For this review, take the finished solid that the model builds, in its own axes (mm). Face numbers are marked on the shaded views. Coordinates: 2 decimals unless noted, no trailing zeros. Loops run counter-clockwise (first coordinate to the right, second up) from the corner with the lowest first, then second, coordinate; pieces in that order, holes last. Notation, with made-up numbers: (22, 13) - (60, 13) arc R19 cw to (60, 35) - close; hole circle Ø3 at (28, 32). An arc over 180 degrees is marked (long way). One line per item, written item: value. Start each with the question number.
1. Take a section at A-A, the plane z = -22.85. State the section outline as (x, y) points (3 decimals), and give its area (3 significant figures).
2. To check wall thickness, follow line 1 (Z direction, x = 5, y = 16.75); line 2 (Z direction, x = 52.95, y = 0.7) (3 decimals); line 3 (X direction, y = 0.7, z = -22.85) (3 decimals). State the ranges of each line that lie inside material, in increasing order. Write a range as from..to.
3. Take a section at B-B, the plane y = 8.5. State the section outline as (x, z) points, and give its area (3 significant figures).
4. The part is to be moulded in two halves that separate along Z. For the marked faces 1, 2, 3 and 4, say which applies: released by +Z, released by -Z, zero draft, split by the parting line, or undercut.
5. Take a section at C-C, the plane x = 7. State the section outline as (y, z) points, and give its area (3 significant figures).
6. Insertion check: pin 1 (2.5 mm diameter, centred on x = 52.95, z = -22.85, fed in from +Y). The pin has a flat end and moves straight along its axis. Give the tip position at first contact, or say it passes through.
```python
from build123d import *

# Parameters (mm, degrees)
SKETCH1_R           = 2.225
BASEPLATE_DEPTH     = 1
BOSS_EXTRUDE4_DEPTH = 21.9


with BuildPart() as part:
    # Sketch1 → BasePlate (new body)
    with BuildSketch(Plane(origin=(0, 0, 0), x_dir=(1, 0, 0), z_dir=(0, 1, 0))):
        with BuildLine():
            Line((5.45, 25.1), (0, 25.1))
            Line((0, 25.1), (0, 45.7))
            Line((0, 45.7), (58.4, 45.7))
            Line((58.4, 45.7), (58.4, 0))
            Line((58.4, 0), (0, 0))
            Line((0, 0), (0, 20.6))
            Line((0, 20.6), (5.45, 20.6))
            ThreePointArc((5.45, 20.6), (7.7, 22.85), (5.45, 25.1))
        make_face()
        with Locations((52.95, 22.85)):
            Circle(SKETCH1_R, mode=Mode.SUBTRACT)
    extrude(amount=BASEPLATE_DEPTH)

    # Sketch2 → Boss-Extrude4 (add)
    with BuildSketch(Plane(origin=(0, 1, 0), x_dir=(1, 0, 0), z_dir=(0, 1, 0))):
        with BuildLine():
            Line((52.95, 27.35), (58.4, 27.35))
            Line((58.4, 27.35), (58.4, 45.7))
            Line((58.4, 45.7), (0, 45.7))
            Line((0, 45.7), (0, 27.35))
            Line((0, 27.35), (5.45, 27.35))
            ThreePointArc((5.45, 27.35), (9.95, 22.85), (5.45, 18.35))
            Line((5.45, 18.35), (0, 18.35))
            Line((0, 18.35), (0, 0))
            Line((0, 0), (58.4, 0))
            Line((58.4, 0), (58.4, 18.35))
            Line((58.4, 18.35), (52.95, 18.35))
            ThreePointArc((52.95, 18.35), (48.45, 22.85), (52.95, 27.35))
        make_face()
    extrude(amount=BOSS_EXTRUDE4_DEPTH)


solid = part.part
```
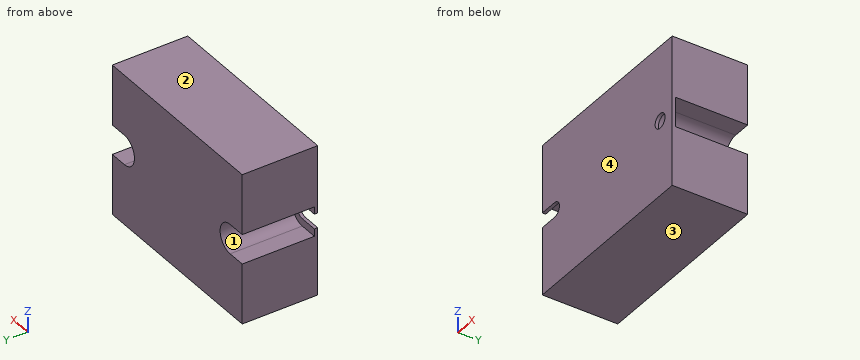
Solutions:
1. outline: (7.7, 0) - (50.725, 0) - (50.725, 1) - (48.45, 1) - (48.45, 22.9) - (9.95, 22.9) - (9.95, 1) - (7.7, 1) - close; (55.175, 0) - (58.4, 0) - (58.4, 1) - (55.175, 1) - close
1. area: 889 mm2
2. line 1: -45.7..-27.35, -18.35..0
2. line 2: -45.7..-25.075, -20.625..0
2. line 3: 7.7..50.725, 55.175..58.4
3. outline: (0, -45.7) - (58.4, -45.7) - (58.4, -27.35) - (52.95, -27.35) arc R4.5 cw to (52.95, -18.35) - (58.4, -18.35) - (58.4, 0) - (0, 0) - (0, -18.35) - (5.45, -18.35) arc R4.5 cw to (5.45, -27.35) - (0, -27.35) - close
3. area: 2,510 mm2
4. face 1: undercut
4. face 2: released by +Z
4. face 3: released by -Z
4. face 4: zero draft
5. outline: (0, -45.7) - (22.9, -45.7) - (22.9, -27.07) - (1, -27.07) - (1, -24.48) - (0, -24.48) - close; (0, -21.22) - (1, -21.22) - (1, -18.63) - (22.9, -18.63) - (22.9, 0) - (0, 0) - close
5. area: 858 mm2
6. pin 1: through
